Model file for the job. Use its own axes, mm. A direction names the side the tool comes from. Round coordinates to 2 decimals unless told otherwise and drop trailing zeros. Write each loop counter-clockwise with the first axis right and the second up, starting at its lowest first coordinate (ties: lowest second). Pieces come first, ordered by that corner, then holes.
```python
from build123d import *

# Parameters (mm, degrees)
BASE_FLANGE1_DEPTH       = 20
EDGE_FLANGE1_START       = -2
EDGE_FLANGE1_DEPTH       = 2
EDGE_FLANGE1_START_2     = -250
EDGE_FLANGE1_2_OUTLINE_W = 2
EDGE_FLANGE1_2_OUTLINE_H = 192
EDGE_FLANGE1_2_DEPTH     = 2.292893219
EDGE_FLANGE1_3_DEPTH     = 2
EDGE_FLANGE1_START_3     = -247
EDGE_FLANGE1_4_DEPTH     = 244
EDGE_FLANGE1_START_4     = 3
EDGE_FLANGE1_5_DEPTH     = 194


with BuildPart() as part:
    # Base-Flange1: sheet metal written as solids
    # Sketch1 → Base-Flange1 (new body)
    with BuildSketch(Plane(origin=(0, 0, 0), x_dir=(0, 0, -1), z_dir=(1, 0, 0))):
        with BuildLine():
            Line((245, 200), (3, 200))
            ThreePointArc((3, 200), (0.878679656, 199.121320344), (0, 197))
            Line((0, 197), (0, 3))
            ThreePointArc((0, 3), (0.878679656, 0.878679656), (3, 0))
            Line((3, 0), (247, 0))
            ThreePointArc((247, 0), (249.121320344, 0.878679656), (250, 3))
            Line((250, 3), (250, 195))
            Line((250, 195), (252, 195))
            Line((252, 195), (252, 3))
            ThreePointArc((252, 3), (250.535533906, -0.535533906), (247, -2))
            Line((247, -2), (3, -2))
            ThreePointArc((3, -2), (-0.535533906, -0.535533906), (-2, 3))
            Line((-2, 3), (-2, 197))
            ThreePointArc((-2, 197), (-0.535533906, 200.535533906), (3, 202))
            Line((3, 202), (245, 202))
            Line((245, 202), (245, 200))
        make_face()
    extrude(amount=BASE_FLANGE1_DEPTH)

    # Edge-Flange1: read off the stored shape, not the designer's step
    # Edge-Flange1 outline → Edge-Flange1 (add)
    with BuildSketch(Plane(origin=(0, 200, 0), x_dir=(0, 0, -1), z_dir=(-1, 0, 0)).offset(EDGE_FLANGE1_START)):
        Polygon((247, 197.707106781), (247, 200), (3, 200), (3, 197.707106781), (19.707106781, 181), (230.292893219, 181), align=None)
        Polygon((2.292893219, 197), (0, 197), (0, 3), (2.292893219, 3), (19, 19.707106781), (19, 180.292893219), align=None)
        Polygon((245, 0), (245, 4.292893219), (230.292893219, 19), (19.707106781, 19), (3, 2.292893219), (3, 0), align=None)
    extrude(amount=EDGE_FLANGE1_DEPTH)

    # Edge-Flange1 2 outline → Edge-Flange1 2 (add)
    with BuildSketch(Plane.XY.offset(EDGE_FLANGE1_START_2)):
        with Locations((1, 99)):
            Rectangle(EDGE_FLANGE1_2_OUTLINE_W, EDGE_FLANGE1_2_OUTLINE_H)
    extrude(amount=EDGE_FLANGE1_2_DEPTH)

    # Edge-Flange1 3 outline → Edge-Flange1 3 (add)
    with BuildSketch(Plane.YZ):
        Polygon((180.292893219, -231), (19.707106781, -231), (3, -247.707106781), (195, -247.707106781), (195, -245.707106781), align=None)
    extrude(amount=EDGE_FLANGE1_3_DEPTH)

    # Edge-Flange1 4 outline → Edge-Flange1 4 (cut)
    with BuildSketch(Plane.XY.offset(EDGE_FLANGE1_START_3)):
        with BuildLine():
            Line((0, -2), (2, -2))
            ThreePointArc((2, -2), (0.585786438, -1.414213562), (0, 0))
            Line((0, 0), (0, -2))
        make_face()
        with BuildLine():
            Line((0, 202), (0, 200))
            ThreePointArc((0, 200), (0.585786438, 201.414213562), (2, 202))
            Line((2, 202), (0, 202))
        make_face()
    extrude(amount=EDGE_FLANGE1_4_DEPTH, mode=Mode.SUBTRACT)

    # Edge-Flange1 5 outline → Edge-Flange1 5 (cut)
    with BuildSketch(Plane(origin=(0, 0, 0), x_dir=(1, 0, 0), z_dir=(0, 1, 0)).offset(EDGE_FLANGE1_START_4)):
        with BuildLine():
            Line((0, -2), (2, -2))
            ThreePointArc((2, -2), (0.585786438, -1.414213562), (0, 0))
            Line((0, 0), (0, -2))
        make_face()
        with BuildLine():
            Line((0, 252), (0, 250))
            ThreePointArc((0, 250), (0.585786438, 251.414213562), (2, 252))
            Line((2, 252), (0, 252))
        make_face()
    extrude(amount=EDGE_FLANGE1_5_DEPTH, mode=Mode.SUBTRACT)


solid = part.part
```
1) Which spindle directions (+Z, -Z, +X, -X, +Y, -Y) get a long thin tool onto all of the face, cutting with end or side? Do faces 1 (the face through (11, 101, 0)), 2 (the face through (0.986, 187.749, -238.457)), 3 (the face through (11, 200, -126)). Say none if no direction does.
2) Cut at A-A on y = 159.5. List the corners of the cut face in (x, z), and give its area (3 significant figures).
3) Wall check: probe 1 along Y at (x, z) = (14.5, -153.5); probe 2 along Z at (x, y) = (4, 30); probe 3 along X at (y, z) = (181.5, -84). Give the ranges that are in metal, low to high.
4) Cut at C-C on x = 15. List the corners of the cut face in (y, z).
5) Pull direction Y, two halves, no side cores. Call faces 4 (the face through (11, 100, -252)), 5 (the face through (7.6, 195, -250.3)), 6 (the face through (1.014, 188.763, -10.529)): released by +Y, released by -Y, zero draft, split by the parting line, or undercut.
6) Flat gauge pins, fed straight in: pin 1 Ø1.6 at (x, z) = (0.5, 1) entering from -Y; pin 2 Ø1 at (x, y) = (1, 66) entering from -Z; pin 3 Ø8 at (y, z) = (23.5, -141.5) entering from +X; pin 4 Ø1.6 at (x, y) = (0.5, -1.5) entering from -Z. Where does each tip first touch, or does it go through?
7) Cut at B-B on z = -87. List the corners of the cut face in (x, y).
Result sheet:
1. face 1: +X
1. face 2: +X, -X
1. face 3: -Z, +X
2. outline: (0, -250) arc R2 ccw to (2, -252) - (20, -252) - (20, -250) - (2, -250) - (2, -231) - (0, -231) - close; (0, -19) - (2, -19) - (2, 0) - (20, 0) - (20, 2) - (2, 2) arc R2 ccw to (0, 0) - close
2. area: 154 mm2
3. probe 1: y = -2 to 0, 200 to 202
3. probe 2: z = -252 to -250, 0 to 2
3. probe 3: x = 0 to 2
4. outline: (-2, -247) arc R5 ccw to (3, -252) - (195, -252) - (195, -250) - (3, -250) arc R3 cw to (0, -247) - (0, -3) arc R3 cw to (3, 0) - (197, 0) arc R3 cw to (200, -3) - (200, -245) - (202, -245) - (202, -3) arc R5 ccw to (197, 2) - (3, 2) arc R5 ccw to (-2, -3) - close
5. face 4: zero draft
5. face 5: released by +Y
5. face 6: undercut
6. pin 1: stops at y = -0.84
6. pin 2: stops at z = -251.94
6. pin 3: passes through
6. pin 4: stops at z = -250.36
7. outline: (0, 0) arc R2 ccw to (2, -2) - (20, -2) - (20, 0) - (2, 0) - (2, 19) - (0, 19) - close; (0, 181) - (2, 181) - (2, 200) - (20, 200) - (20, 202) - (2, 202) arc R2 ccw to (0, 200) - close
